from build123d import *

# Parameters (mm, degrees)
EXTRUDE_1_DEPTH                    = 2.55
CUT_EXTRUDE_1_DEPTH                = 9.2
EXTRUDE_2_DEPTH                    = 3.8
SKETCH_4_W                         = 5.63
SKETCH_4_H                         = 1
CUT_EXTRUDE_2_DEPTH                = 3.8
CUT_EXTRUDE_3_REACH                = 16.048
CHAMFER_1_SIZE                     = 0.5
EXTRUDE_START                      = -3.6
SKETCH_6_W                         = 0.64
SKETCH_6_H                         = 0.64
EXTRUDE_3_DEPTH                    = 11.7
CHAMFER_2_SIZE                     = 0.2
PATTERN_LINEAR_1_COUNT             = 2
PATTERN_LINEAR_1_PITCH             = 2.54
CHAMFER_2_OF_PATTERN_LINEAR_1_SIZE = 0.2


with BuildPart() as part:
    # Эскиз1 → Бобышка-Вытянуть1 (new, symmetric)
    with BuildSketch(Plane(origin=(0, 0, 0), x_dir=(1, 0, 0), z_dir=(0, 1, 0))):
        Polygon((-2.415, -0.3), (2.415, -0.3), (2.415, 0), (3.115, 0), (3.115, -0.3), (3.815, -0.3), (3.815, -11.8), (-3.815, -11.8), (-3.815, -0.3), (-3.115, -0.3), (-3.115, 0), (-2.415, 0), align=None)
    extrude(amount=EXTRUDE_1_DEPTH, both=True)

    # Эскиз2 → Вырез-Вытянуть1 (cut)
    with BuildSketch(Plane.XY.offset(11.8)):
        Polygon((-2.815, 1.55), (-2.815, -1.55), (-0.6, -1.55), (-0.6, -2.55), (0.6, -2.55), (0.6, -1.55), (2.815, -1.55), (2.815, 1.55), (1.5, 1.55), (1.5, 2.55), (-1.5, 2.55), (-1.5, 1.55), align=None)
    extrude(amount=-CUT_EXTRUDE_1_DEPTH, mode=Mode.SUBTRACT)

    # Эскиз3 → Бобышка-Вытянуть2 (add)
    with BuildSketch(Plane.XY.offset(11.8)):
        Polygon((-3.815, 2.55), (-3.815, 4.05), (3.815, 4.05), (3.815, 2.55), (2.815, 2.55), (2.815, 3.05), (-2.815, 3.05), (-2.815, 2.55), align=None)
    extrude(amount=-EXTRUDE_2_DEPTH)

    # Эскиз4 → Вырез-Вытянуть2 (cut)
    with BuildSketch(Plane.XY.offset(11.8)):
        with Locations((0, 2.05)):
            Rectangle(SKETCH_4_W, SKETCH_4_H)
    extrude(amount=-CUT_EXTRUDE_2_DEPTH, mode=Mode.SUBTRACT)

    # Эскиз5 → Вырез-Вытянуть3 (cut, up to next)
    with BuildSketch(Plane(origin=(0, 4.05, 0), x_dir=(1, 0, 0), z_dir=(0, 1, 0)), mode=Mode.PRIVATE) as cut_extrude_3_sk1:
        with BuildLine():
            Line((2.815, -8), (2.815, -9.8))
            ThreePointArc((2.815, -9.8), (2.668553391, -10.153553391), (2.315, -10.3))
            Line((2.315, -10.3), (-2.315, -10.3))
            ThreePointArc((-2.315, -10.3), (-2.668553391, -10.153553391), (-2.815, -9.8))
            Line((-2.815, -9.8), (-2.815, -8))
            Line((-2.815, -8), (2.815, -8))
        make_face()
    cut_extrude_3_tool1 = extrude(cut_extrude_3_sk1.sketch, amount=-CUT_EXTRUDE_3_REACH, mode=Mode.PRIVATE) & part.part
    add(cut_extrude_3_tool1.solids().sort_by_distance((0, 4.05, 9.141324))[0], mode=Mode.SUBTRACT)

    # Фаска1
    chamfer_1_edges = [part.edges().sort_by_distance(p)[0] for p in [
        (-2.1575, 1.55, 8),
        (2.1575, 1.55, 8),
        (-2.815, 0.75, 11.8),
        (-1.7075, -1.55, 11.8),
        (1.7075, -1.55, 11.8),
        (2.815, 0.75, 11.8),
        (0, 3.05, 11.8),
    ]]
    chamfer(chamfer_1_edges, length=CHAMFER_1_SIZE)

    # Эскиз6 → Бобышка-Вытянуть3 (add)
    with BuildSketch(Plane.XY.offset(0.3).offset(EXTRUDE_START)):
        with Locations((1.27, 0)):
            Rectangle(SKETCH_6_W, SKETCH_6_H)
    extrude_3 = extrude(amount=EXTRUDE_3_DEPTH)

    # Фаска2
    chamfer_2_edges = [part.edges().sort_by_distance(p)[0] for p in [
        (1.27, 0.32, 8.4),
        (1.59, 0, 8.4),
        (1.27, -0.32, 8.4),
        (0.95, 0, 8.4),
        (0.95, 0, -3.3),
        (1.27, 0.32, -3.3),
        (1.59, 0, -3.3),
        (1.27, -0.32, -3.3),
    ]]
    chamfer(chamfer_2_edges, length=CHAMFER_2_SIZE)

    # Линейный массив1: Бобышка-Вытянуть3 ×2
    with Locations(*[(-i * PATTERN_LINEAR_1_PITCH, 0, 0) for i in range(1, PATTERN_LINEAR_1_COUNT)]):
        add(extrude_3)

    # Фаска2 of Линейный массив1
    chamfer_2_of_pattern_linear_1_edges = [part.edges().sort_by_distance(p)[0] for p in [
        (-1.27, 0.32, 8.4),
        (-0.95, 0, 8.4),
        (-1.27, -0.32, 8.4),
        (-1.59, 0, 8.4),
        (-1.59, 0, -3.3),
        (-1.27, 0.32, -3.3),
        (-0.95, 0, -3.3),
        (-1.27, -0.32, -3.3),
    ]]
    chamfer(chamfer_2_of_pattern_linear_1_edges, length=CHAMFER_2_OF_PATTERN_LINEAR_1_SIZE)


solid = part.part
Source: CAD feature listing. Evaluate the final solid. Frame: model axes, mm. A direction names the side the tool comes from. Round coordinates to 2 decimals unless told otherwise and drop trailing zeros. Write each loop counter-clockwise with the first axis right and the second up, starting at its lowest first coordinate (ties: lowest second). Pieces come first, ordered by that corner, then holes. Notation, with made-up numbers: (24, 0) - (67, 0) arc R25 cw to (67, 21) - close; hole circle Ø7 at (26.5, 59.5). An arc over 180 degrees is marked (long way). Use CSV: the item, a comma, the result in double quotes. Start each with the question number.
(1) Cut plane B-B, the plane z = 5.25. Return loops of the section in (x, y) (3 decimals), and give its area (3 significant figures).
(2) Mould query, pull axis Y, two halves, no side actions, for faces 1 (the face through (0, 4.05, 11)), 2 (the face through (-2, 1.55, 5)), 3 (the face through (3.815, 0, 6)). Classes: pulls with the +Y half, pulls with the -Y half, needs draft (parallel to the pull), parting line crosses it, or undercut.
(3) Cut plane C-C, the plane z = -2.25. Return loops of the section in (x, y).
(4) Set-up query: faces 4 (the face through (-2, -1.55, 7)), 5 (the face through (-1.5, 2, 5)), 6 (the face through (0, 2.55, 2)), 7 (the face through (-0.6, -2, 7)). Return all of +Z, -Z, +X, -X, +Y, -Y with unobstructed straight access to the full face (end or side cutting, diameter ignored); none if empty.
(5) Material intervals for probe 1 along X at (y, z) = (-0.75, 5.5) (3 decimals); probe 2 along X at (y, z) = (-2, 11.25) (3 decimals); probe 3 along Y at (x, z) = (-1, 3.75), sorted ascending. Write a range as [from, to].
(6) Cut plane D-D, the plane y = 1.75. Return loops of the section in (x, z) (3 decimals), and give its area (3 significant figures).
(7) First-contact query: pin 1 Ø2.5 at (x, z) = (0, 3.5) entering from +Y; pin 2 Ø3 at (x, y) = (0.5, 1.5) entering from +Z. Flat tips, straight axial feed; report the tip coordinate or a pass-through.
(8) Cut plane A-A, the plane x = 2. Return loops of the section in (y, z).
Geometry says:
1,outline,"(-3.815, -2.55) - (-0.6, -2.55) - (-0.6, -1.55) - (-2.815, -1.55) - (-2.815, 1.55) - (-1.5, 1.55) - (-1.5, 2.55) - (-3.815, 2.55) - close; (-1.59, -0.32) - (-0.95, -0.32) - (-0.95, 0.32) - (-1.59, 0.32) - close; (0.6, -2.55) - (3.815, -2.55) - (3.815, 2.55) - (1.5, 2.55) - (1.5, 1.55) - (2.815, 1.55) - (2.815, -1.55) - (0.6, -1.55) - close; (0.95, -0.32) - (1.59, -0.32) - (1.59, 0.32) - (0.95, 0.32) - close"
1,area,"18.1 mm²"
2,face 1,"pulls with the +Y half"
2,face 2,"undercut"
2,face 3,"needs draft"
3,outline,"(-1.59, -0.32) - (-0.95, -0.32) - (-0.95, 0.32) - (-1.59, 0.32) - close; (0.95, -0.32) - (1.59, -0.32) - (1.59, 0.32) - (0.95, 0.32) - close"
4,face 4,"+Z"
4,face 5,"+Z, +Y"
4,face 6,"-Z, +X, -X, +Y"
4,face 7,"+Z, -Y"
5,probe 1,"[-3.815, -2.815], [2.815, 3.815]"
5,probe 2,"[-3.815, -0.6], [0.6, 3.815]"
5,probe 3,"[-2.55, -1.55], [-0.32, 0.32]"
6,outline,"(-3.815, 0.3) - (-3.115, 0.3) - (-3.115, 0) - (-2.415, 0) - (-2.415, 0.3) - (2.415, 0.3) - (2.415, 0) - (3.115, 0) - (3.115, 0.3) - (3.815, 0.3) - (3.815, 11.8) - (3.315, 11.8) - (2.815, 11.3) - (2.815, 7.7) - (1.5, 7.7) - (1.5, 2.6) - (-1.5, 2.6) - (-1.5, 7.7) - (-2.815, 7.7) - (-2.815, 11.3) - (-3.315, 11.8) - (-3.815, 11.8) - close"
6,area,"49.5 mm²"
7,pin 1,"y = 2.55"
7,pin 2,"z = 8.38"
8,outline,"(-2.55, 0.3) - (2.55, 0.3) - (2.55, 8) - (2.05, 8) - (1.55, 7.5) - (1.55, 2.6) - (-1.55, 2.6) - (-1.55, 11.3) - (-2.05, 11.8) - (-2.55, 11.8) - close; (3.05, 10.3) - (4.05, 10.3) - (4.05, 11.8) - (3.55, 11.8) - (3.05, 11.3) - close"
